Source: CAD feature listing. Evaluate the final solid. Frame: model axes, mm. A direction names the side the tool comes from. Round coordinates to 2 decimals unless told otherwise and drop trailing zeros. Loops run counter-clockwise (first coordinate to the right, second up) from the corner with the lowest first, then second, coordinate; pieces in that order, holes last. Notation, with made-up numbers: M 45,51.25 L 66,51.25 A13 cw 66,72.25 Z; hole C 61,-34.5 d8. An arc over 180 degrees is marked long. Answer as a JSON object with one key per item and string values.
from build123d import *

# Parameters (mm, degrees)
EXTRUDE_1_DEPTH          = 15
CUT_EXTRUDE_1_DEPTH      = 328.223165439
CUT_EXTRUDE_1_DEPTH_BACK = 328.223165439
SKETCH_3_R               = 16
CUT_EXTRUDE_2_DEPTH      = 12.5


with BuildPart() as part:
    # Эскиз1 → Бобышка-Вытянуть1 (new, symmetric)
    with BuildSketch(Plane.XY):
        with BuildLine():
            Line((1.166666667, 34.980550151), (300.833333333, 24.986107251))
            ThreePointArc((300.833333333, 24.986107251), (325, 0), (300.833333333, -24.986107251))
            Line((300.833333333, -24.986107251), (1.166666667, -34.980550151))
            ThreePointArc((1.166666667, -34.980550151), (-35, 0), (1.166666667, 34.980550151))
        make_face()
    extrude(amount=EXTRUDE_1_DEPTH, both=True)

    # Эскиз3 → Вырез-Вытянуть1 (cut, two sides: drawn at the far end of the back side and taken through both)
    with BuildSketch(Plane.XY.offset(-CUT_EXTRUDE_1_DEPTH_BACK)):
        Circle(SKETCH_3_R)
    extrude(amount=CUT_EXTRUDE_1_DEPTH + CUT_EXTRUDE_1_DEPTH_BACK, mode=Mode.SUBTRACT)

    # Эскиз4 → Вырез-Вытянуть2 (cut, symmetric)
    with BuildSketch(Plane.XY):
        with BuildLine():
            Line((230, 23.346307109), (210, 24.013344455))
            Line((210, 24.013344455), (210, 28.015568531))
            Line((210, 28.015568531), (141.166666667, 30.31128873))
            Line((141.166666667, 30.31128873), (141.166666667, 26.309064654))
            Line((141.166666667, 26.309064654), (121.166666667, 26.976102))
            Line((121.166666667, 26.976102), (121.166666667, 30.978326076))
            Line((121.166666667, 30.978326076), (21.166666667, 34.313512805))
            Line((21.166666667, 34.313512805), (21.166666667, 30.31128873))
            Line((21.166666667, 30.31128873), (1.033333333, 30.982772991))
            ThreePointArc((1.033333333, 30.982772991), (-31, 0), (1.033333333, -30.982772991))
            Line((1.033333333, -30.982772991), (21.166666667, -30.31128873))
            Line((21.166666667, -30.31128873), (21.166666667, -34.313512805))
            Line((21.166666667, -34.313512805), (121.166666667, -30.978326076))
            Line((121.166666667, -30.978326076), (121.166666667, -26.976102))
            Line((121.166666667, -26.976102), (141.166666667, -26.309064654))
            Line((141.166666667, -26.309064654), (141.166666667, -30.31128873))
            Line((141.166666667, -30.31128873), (210, -28.015568531))
            Line((210, -28.015568531), (210, -24.013344455))
            Line((210, -24.013344455), (230, -23.346307109))
            Line((230, -23.346307109), (230, -27.348531185))
            Line((230, -27.348531185), (300.833333333, -24.986107251))
            ThreePointArc((300.833333333, -24.986107251), (325, 0), (300.833333333, 24.986107251))
            Line((300.833333333, 24.986107251), (230, 27.348531185))
            Line((230, 27.348531185), (230, 23.346307109))
        make_face()
    extrude(amount=CUT_EXTRUDE_2_DEPTH, both=True, mode=Mode.SUBTRACT)


solid = part.part
Item 1: Contact query for flat-ended pins moving along their axis: pin 1 Ø2 at (y, z) = (29.5, -5.5) entering from -X; pin 2 Ø4.5 at (y, z) = (31.5, 5) entering from +X; pin 3 Ø3 at (y, z) = (-27.5, 0.5) entering from +X; pin 4 Ø12 at (x, z) = (155, -3.5) entering from +Y. Output: stop coordinate, or through.
Answer sheet:
{"pin 1": "stops at x = -20.32", "pin 2": "stops at x = 141.17", "pin 3": "stops at x = 230", "pin 4": "passes through"}
Item 2: Access query for faces 1 (the flat face through (148, 0, 15)), 2 (the flat face through (145, 0, -12.5)). Directions: +Z, -Z, +X, -X, +Y, -Y. A direction counts if a zero-diameter tool reaches every point of the face in a straight line with its end or side. Return the directions, or none.
Answer sheet:
{"face 1": "+Z, +X, -X, +Y, -Y", "face 2": "none"}
Item 3: Section A-A on y = 0. Return the cut outline in (x, z).
Answer sheet:
{"outline": "M -35,-15 L -16,-15 L -16,-12.5 L -31,-12.5 L -31,12.5 L -16,12.5 L -16,15 L -35,15 Z; M 16,-15 L 325,-15 L 325,-12.5 L 16,-12.5 Z; M 16,12.5 L 325,12.5 L 325,15 L 16,15 Z"}
Item 4: Line query: probe 1 along Y at (x, z) = (0, -13); probe 2 along Z at (x, y) = (284, -7); probe 3 along X at (y, z) = (0, 13.9). Output: solid intervals per line, ascending. Write a range as from..to.
Answer sheet:
{"probe 1": "y = -35..-16, 16..35", "probe 2": "z = -15..-12.5, 12.5..15", "probe 3": "x = -35..-16, 16..325"}
Item 5: Section B-B on z = -1.75. Return the cut outline in (x, y).
Answer sheet:
{"outline": "M 1.03,-30.98 A31 cw long 1.03,30.98 L 21.17,30.31 L 21.17,34.31 L 1.17,34.98 A35 ccw long 1.17,-34.98 L 21.17,-34.31 L 21.17,-30.31 Z; M 121.17,-30.98 L 141.17,-30.31 L 141.17,-26.31 L 121.17,-26.98 Z; M 121.17,26.98 L 141.17,26.31 L 141.17,30.31 L 121.17,30.98 Z; M 210,-28.02 L 230,-27.35 L 230,-23.35 L 210,-24.01 Z; M 210,24.01 L 230,23.35 L 230,27.35 L 210,28.02 Z"}
Item 6: Section D-D on x = 223. Return the cut outline in (y, z).
Answer sheet:
{"outline": "M -27.58,-15 L 27.58,-15 L 27.58,15 L -27.58,15 Z; hole M -23.58,-12.5 L 23.58,-12.5 L 23.58,12.5 L -23.58,12.5 Z"}
Item 7: Section C-C on x = 111.5. Return the cut outline in (y, z).
Answer sheet:
{"outline": "M -31.3,-15 L 31.3,-15 L 31.3,-12.5 L -31.3,-12.5 Z; M -31.3,12.5 L 31.3,12.5 L 31.3,15 L -31.3,15 Z"}
Item 8: Pull-direction query (X, two-part tool) for faces 3 (the cylindrical face through (-30.992, 0.696, 0.175)), 4 (the cylindrical face through (324.994, 0.538, 13.768)), 5 (the flat face through (148, 0, -15)); classes: pulls with the +X half, pulls with the -X half, needs draft (parallel to the pull), parting line crosses it, or undercut.
Answer sheet:
{"face 3": "undercut", "face 4": "pulls with the +X half", "face 5": "needs draft"}
